```python
from build123d import *

# Parameters (mm, degrees)
SKETCH1_R           = 42
SKETCH1_R_2         = 12
SKETCH1_R_3         = 1
BOSS_EXTRUDE1_DEPTH = 5


with BuildPart() as part:
    # Sketch1 → Boss-Extrude1 (new body)
    with BuildSketch(Plane(origin=(0, 0, 0), x_dir=(1, 0, 0), z_dir=(0, 1, 0))):
        with Locations(Location((0, 0, 0), (0, 0, 270))):
            Circle(SKETCH1_R)
        with Locations(Location((0, 0, 0), (0, 0, 270))):
            Circle(SKETCH1_R_2, mode=Mode.SUBTRACT)
        with Locations(Location((35, 0, 0), (0, 0, 270))):
            Circle(SKETCH1_R_3, mode=Mode.SUBTRACT)
        with Locations(Location((32.335783638, -13.393920133, 0), (0, 0, 270))):
            Circle(SKETCH1_R_3, mode=Mode.SUBTRACT)
        with Locations(Location((24.748737342, -24.748737342, 0), (0, 0, 270))):
            Circle(SKETCH1_R_3, mode=Mode.SUBTRACT)
        with Locations(Location((13.393920133, -32.335783638, 0), (0, 0, 270))):
            Circle(SKETCH1_R_3, mode=Mode.SUBTRACT)
        with Locations(Location((0, -35, 0), (0, 0, 270))):
            Circle(SKETCH1_R_3, mode=Mode.SUBTRACT)
        with Locations(Location((-13.393920133, -32.335783638, 0), (0, 0, 270))):
            Circle(SKETCH1_R_3, mode=Mode.SUBTRACT)
        with Locations(Location((-24.748737342, -24.748737342, 0), (0, 0, 270))):
            Circle(SKETCH1_R_3, mode=Mode.SUBTRACT)
        with Locations(Location((-32.335783638, -13.393920133, 0), (0, 0, 270))):
            Circle(SKETCH1_R_3, mode=Mode.SUBTRACT)
        with Locations(Location((-35, 0, 0), (0, 0, 270))):
            Circle(SKETCH1_R_3, mode=Mode.SUBTRACT)
        with Locations(Location((-32.335783638, 13.393920133, 0), (0, 0, 270))):
            Circle(SKETCH1_R_3, mode=Mode.SUBTRACT)
        with Locations(Location((-24.748737342, 24.748737342, 0), (0, 0, 270))):
            Circle(SKETCH1_R_3, mode=Mode.SUBTRACT)
        with Locations(Location((-13.393920133, 32.335783638, 0), (0, 0, 270))):
            Circle(SKETCH1_R_3, mode=Mode.SUBTRACT)
        with Locations(Location((0, 35, 0), (0, 0, 270))):
            Circle(SKETCH1_R_3, mode=Mode.SUBTRACT)
        with Locations(Location((13.393920133, 32.335783638, 0), (0, 0, 270))):
            Circle(SKETCH1_R_3, mode=Mode.SUBTRACT)
        with Locations(Location((24.748737342, 24.748737342, 0), (0, 0, 270))):
            Circle(SKETCH1_R_3, mode=Mode.SUBTRACT)
        with Locations(Location((32.335783638, 13.393920133, 0), (0, 0, 270))):
            Circle(SKETCH1_R_3, mode=Mode.SUBTRACT)
    extrude(amount=BOSS_EXTRUDE1_DEPTH)


solid = part.part
```
The listing builds one solid part. Answer for the finished solid, in the listing's coordinates (mm). Round coordinates to 2 decimals unless told otherwise and drop trailing zeros. Loops run counter-clockwise (first coordinate to the right, second up) from the corner with the lowest first, then second, coordinate; pieces in that order, holes last.
Q1. Section B-B, the plane z = 0 is taken. Determine the outline of the cut face in (x, y), then the cut area to 3 significant figures.
Q2. For a pull along X with two mould halves and no side action, classify faces 1 (the face through (24.79, 2.46, 23.75)), 2 (the face through (12.62, 2.46, 40.06)), 3 (the face through (-9, 0, 9)), 4 (the face through (-31.344, 2.465, 13.264)) as released by +X, released by -X, zero draft, split by the parting line, or undercut.
Q3. Section A-A, the plane x = 0 is taken. Determine the outline of the cut face in (y, z), then the cut area to 3 significant figures.
Q4. Section D-D, the plane x = -35 is taken. Determine the outline of the cut face in (y, z), then the cut area to 3 significant figures.
Q5. Section C-C, the plane z = -10.5 is taken. Determine the outline of the cut face in (x, y), then the cut area to 3 significant figures.
Q6. Given pin 1 Ø1.6 at (x, z) = (-32.34, -13.39) entering from +Y; pin 2 Ø1 at (x, y) = (19, 4) entering from -Z; pin 3 Ø1.5 at (x, y) = (-23.5, 4) entering from +Z; pin 4 Ø2 at (y, z) = (4.5, 32) entering from -X, each flat-ended and moving along its own axis, determine where each tip first touches the part or whether it passes through.
Q7. Find the intervals of material crossed by line 1 (X direction, y = 1.3, z = 0); line 2 (Z direction, x = -32.5, y = 1.3); line 3 (X direction, y = 2.7, z = 14), in increasing order.
Completed:
1. outline: (-42, 0) - (-36, 0) - (-36, 5) - (-42, 5) - close; (-34, 0) - (-12, 0) - (-12, 5) - (-34, 5) - close; (12, 0) - (34, 0) - (34, 5) - (12, 5) - close; (36, 0) - (42, 0) - (42, 5) - (36, 5) - close
1. area: 280 mm2
2. face 1: undercut
2. face 2: split by the parting line
2. face 3: zero draft
2. face 4: undercut
3. outline: (0, -42) - (5, -42) - (5, -36) - (0, -36) - close; (0, -34) - (5, -34) - (5, -12) - (0, -12) - close; (0, 12) - (5, 12) - (5, 34) - (0, 34) - close; (0, 36) - (5, 36) - (5, 42) - (0, 42) - close
3. area: 280 mm2
4. outline: (0, -23.22) - (5, -23.22) - (5, -1) - (0, -1) - close; (0, 1) - (5, 1) - (5, 23.22) - (0, 23.22) - close
4. area: 222 mm2
5. outline: (-40.67, 0) - (-5.81, 0) - (-5.81, 5) - (-40.67, 5) - close; (5.81, 0) - (40.67, 0) - (40.67, 5) - (5.81, 5) - close
5. area: 349 mm2
6. pin 1: passes through
6. pin 2: stops at z = -37.71
6. pin 3: stops at z = 35.3
6. pin 4: stops at x = -28.34
7. line 1: x = -42 to -36, -34 to -12, 12 to 34, 36 to 42
7. line 2: z = -26.6 to -14.38, -12.41 to 12.41, 14.38 to 26.6
7. line 3: x = -39.6 to -33.13, -31.54 to 31.54, 33.13 to 39.6
